CAD build for the part. Positions are in the model's coordinates, mm. Face numbers are marked on the shaded views. A direction names the side the tool comes from. Give positions to 0.01 mm unless a question says otherwise; leave off trailing zeros. Order: outer loops, then holes, each group sorted by start corner. A loop starts at its lowest first (then second) coordinate and runs counter-clockwise, first axis right, second up.
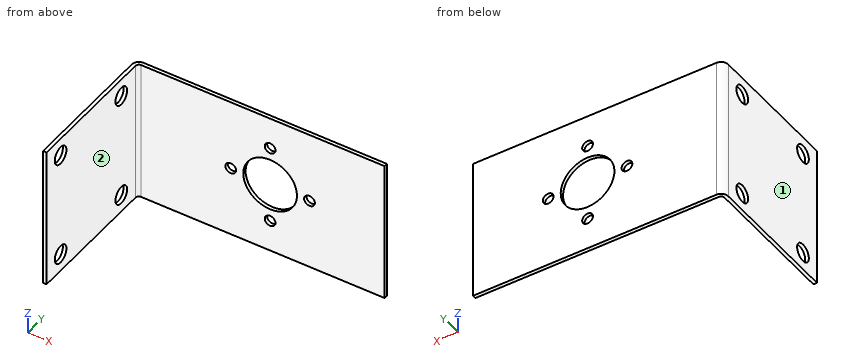
from build123d import *

# Parameters (mm, degrees)
BASE_FLANGE1_DEPTH = 40
CUT_EXTRUDE1_REACH = 92
SKETCH6_R          = 7.5
SKETCH7_R          = 1.5
CUT_EXTRUDE2_DEPTH = 91
CUT_EXTRUDE3_REACH = 92
SKETCH8_R          = 2.5


# Sheet-metal steps are written as plain solids
with BuildPart() as part:
    # Sketch1 → Base-Flange1 (new body)
    with BuildSketch(Plane.XY):
        with BuildLine():
            Line((0, 0), (0, 38))
            ThreePointArc((0, 38), (0.585786438, 39.414213562), (2, 40))
            Line((2, 40), (70, 40))
            Line((70, 40), (70, 39))
            Line((70, 39), (2, 39))
            ThreePointArc((2, 39), (1.292893219, 38.707106781), (1, 38))
            Line((1, 38), (1, 0))
            Line((1, 0), (0, 0))
        make_face()
    extrude(amount=BASE_FLANGE1_DEPTH)

    # Sketch6 → Cut-Extrude1 (cut, up to next)
    with BuildSketch(Plane(origin=(0, 40, 0), x_dir=(1, 0, 0), z_dir=(0, 1, 0)), mode=Mode.PRIVATE) as cut_extrude1_sk1:
        with Locations(Location((38, -20, 0), (0, 0, 270))):
            Circle(SKETCH6_R)
    cut_extrude1_tool1 = extrude(cut_extrude1_sk1.sketch, amount=-CUT_EXTRUDE1_REACH, mode=Mode.PRIVATE) & part.part
    add(cut_extrude1_tool1.solids().sort_by_distance((38, 40, 20))[0], mode=Mode.SUBTRACT)

    # Sketch7 → Cut-Extrude2 (cut, through all)
    with BuildSketch(Plane(origin=(0, 40, 0), x_dir=(1, 0, 0), z_dir=(0, 1, 0))):
        with Locations(Location((49, -20, 0), (0, 0, 270))):
            Circle(SKETCH7_R)
        with Locations(Location((38, -31, 0), (0, 0, 270))):
            Circle(SKETCH7_R)
        with Locations(Location((27, -20, 0), (0, 0, 270))):
            Circle(SKETCH7_R)
        with Locations(Location((38, -9, 0), (0, 0, 270))):
            Circle(SKETCH7_R)
    extrude(amount=-CUT_EXTRUDE2_DEPTH, mode=Mode.SUBTRACT)

    # Sketch8 → Cut-Extrude3 (cut, up to next)
    with BuildSketch(Plane.ZY, mode=Mode.PRIVATE) as cut_extrude3_sk1:
        with Locations((5, 32)):
            Circle(SKETCH8_R)
    cut_extrude3_tool1 = extrude(cut_extrude3_sk1.sketch, amount=-CUT_EXTRUDE3_REACH, mode=Mode.PRIVATE) & part.part
    # Sketch8 → Cut-Extrude3 (cut, up to next)
    with BuildSketch(Plane.ZY, mode=Mode.PRIVATE) as cut_extrude3_sk2:
        with Locations((5, 6)):
            Circle(SKETCH8_R)
    cut_extrude3_tool2 = extrude(cut_extrude3_sk2.sketch, amount=-CUT_EXTRUDE3_REACH, mode=Mode.PRIVATE) & part.part
    # Sketch8 → Cut-Extrude3 (cut, up to next)
    with BuildSketch(Plane.ZY, mode=Mode.PRIVATE) as cut_extrude3_sk3:
        with Locations((35, 6)):
            Circle(SKETCH8_R)
    cut_extrude3_tool3 = extrude(cut_extrude3_sk3.sketch, amount=-CUT_EXTRUDE3_REACH, mode=Mode.PRIVATE) & part.part
    # Sketch8 → Cut-Extrude3 (cut, up to next)
    with BuildSketch(Plane.ZY, mode=Mode.PRIVATE) as cut_extrude3_sk4:
        with Locations((35, 32)):
            Circle(SKETCH8_R)
    cut_extrude3_tool4 = extrude(cut_extrude3_sk4.sketch, amount=-CUT_EXTRUDE3_REACH, mode=Mode.PRIVATE) & part.part
    add(cut_extrude3_tool1.solids().sort_by_distance((0, 32, 5))[0], mode=Mode.SUBTRACT)
    add(cut_extrude3_tool2.solids().sort_by_distance((0, 6, 5))[0], mode=Mode.SUBTRACT)
    add(cut_extrude3_tool3.solids().sort_by_distance((0, 6, 35))[0], mode=Mode.SUBTRACT)
    add(cut_extrude3_tool4.solids().sort_by_distance((0, 32, 35))[0], mode=Mode.SUBTRACT)


solid = part.part
1. Saw through at A-A on y = 32. Give the cut face in (x, z).
2. Saw through at C-C on x = 27. Give the cut face in (y, z).
3. Pin check, flat tips, straight feed: P1, Ø11.5, axis at y = 10, z = 29, coming from the +X side; P2, Ø3.5, axis at x = 38, z = 31, coming from the -Y side; P3, Ø2.5, axis at x = 38, z = 9, coming from the +Y side. Stop position of each tip, or through.
4. Saw through at D-D on z = 35. Give the cut face in (x, y), plus the area to 3 significant figures.
5. Saw through at B-B on z = 20. Give the cut face in (x, y).
6. Wall check: line 1 (X direction, y = 32.5, z = 15); line 2 (Y direction, x = 58, z = 19). Give the ranges that are in metal, low to high.
7. 3-axis set-ups, long thin cutter, end or side, ignore diameter. For the marked faces 1 and 2: which of +Z, -Z, +X, -X, +Y, -Y reach the whole face in a straight line?
Reported:
1. outline: (0, 0) - (1, 0) - (1, 2.5) - (0, 2.5) - close; (0, 7.5) - (1, 7.5) - (1, 32.5) - (0, 32.5) - close; (0, 37.5) - (1, 37.5) - (1, 40) - (0, 40) - close
2. outline: (39, 0) - (40, 0) - (40, 18.5) - (39, 18.5) - close; (39, 21.5) - (40, 21.5) - (40, 40) - (39, 40) - close
3. P1: stops at x = 1
3. P2: stops at y = 39
3. P3: passes through
4. outline: (0, 0) - (1, 0) - (1, 3.5) - (0, 3.5) - close; (0, 8.5) - (1, 8.5) - (1, 29.5) - (0, 29.5) - close; (0, 34.5) - (1, 34.5) - (1, 38) arc R1 cw to (2, 39) - (70, 39) - (70, 40) - (2, 40) arc R2 ccw to (0, 38) - close
4. area: 98.4 mm2
5. outline: (0, 0) - (1, 0) - (1, 38) arc R1 cw to (2, 39) - (25.5, 39) - (25.5, 40) - (2, 40) arc R2 ccw to (0, 38) - close; (28.5, 39) - (30.5, 39) - (30.5, 40) - (28.5, 40) - close; (45.5, 39) - (47.5, 39) - (47.5, 40) - (45.5, 40) - close; (50.5, 39) - (70, 39) - (70, 40) - (50.5, 40) - close
6. line 1: x = 0 to 1
6. line 2: y = 39 to 40
7. face 1: +Z, -Z, -X, +Y, -Y
7. face 2: +Z, -Z, +X, -Y
